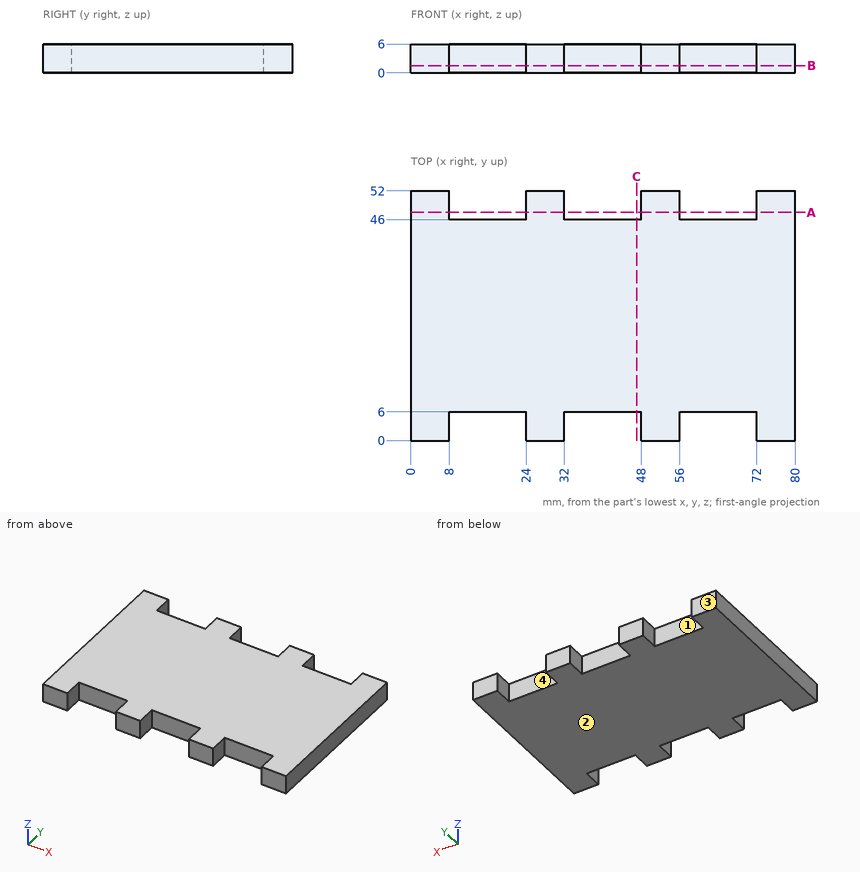
Can you work these out from the drawing? Everything is in mm from the part's minimum corner. A direction names the side the tool comes from. Round coordinates to 2 decimals unless told otherwise and drop trailing zeros. Loops run counter-clockwise (first coordinate to the right, second up) from the corner with the lowest first, then second, coordinate; pieces in that order, holes last. Notation, with made-up numbers: (22, 16) - (58, 16) arc R23 ccw to (58, 36) - close; hole circle Ø5 at (-24, -22.5). An arc over 180 degrees is marked (long way). Answer in a Markdown table with one row per item. Add a question column.
Q1. Which directions (+Z, -Z, +X, -X, +Y, -Y) give clear straight access to the entire face, cutting with the end or side of a thin tool? Please do the marked faces 3 and 4.
Q2. I need wall thicknesses on L1, parallel to X at y = 4, z = 2.4; L2, parallel to Y at x = 62, z = 3.85. Which ranges of each line are inside material? Lowest first, please.
Q3. I want a section at C-C on x = 47. List the corners of the cut face in (y, z) for me.
Q4. I want a section at A-A on y = 47.5. List the corners of the cut face in (x, z) for me.
Q5. I want a section at B-B on z = 1.5. List the corners of the cut face in (x, y) for me, and give its area (3 significant figures).
Q6. We'd pull the mould along X, two halves only. Please class the marked faces 1 and 2: pulls with the +X half, pulls with the -X half, needs draft (parallel to the pull), parting line crosses it, or undercut.
Q7. For pin 1 Ø1.8 at (x, z) = (17.5, 2.5) entering from +Y; pin 2 Ø1.8 at (x, z) = (16, 3) entering from -Y, each with a flat end and sliding along its axis, tell me the tip position at first contact or that it passes through.
A:
| question | item | result |
|---|---|---|
| 1 | face 3 | +Z, -Z, +X, -X, +Y |
| 1 | face 4 | +Z, -Z, +Y |
| 2 | L1 | 0 to 8, 24 to 32, 48 to 56, 72 to 80 |
| 2 | L2 | 6 to 46 |
| 3 | outline | (6, 0) - (46, 0) - (46, 6) - (6, 6) - close |
| 4 | outline | (0, 0) - (8, 0) - (8, 6) - (0, 6) - close; (24, 0) - (32, 0) - (32, 6) - (24, 6) - close; (48, 0) - (56, 0) - (56, 6) - (48, 6) - close; (72, 0) - (80, 0) - (80, 6) - (72, 6) - close |
| 5 | outline | (0, 0) - (8, 0) - (8, 6) - (24, 6) - (24, 0) - (32, 0) - (32, 6) - (48, 6) - (48, 0) - (56, 0) - (56, 6) - (72, 6) - (72, 0) - (80, 0) - (80, 52) - (72, 52) - (72, 46) - (56, 46) - (56, 52) - (48, 52) - (48, 46) - (32, 46) - (32, 52) - (24, 52) - (24, 46) - (8, 46) - (8, 52) - (0, 52) - close |
| 5 | area | 3,580 mm^2 |
| 6 | face 1 | undercut |
| 6 | face 2 | needs draft |
| 7 | pin 1 | y = 46 |
| 7 | pin 2 | y = 6 |
